Read the model definition and answer for the solid it produces. Units are mm, in the model's axes. Round coordinates to 2 decimals unless told otherwise and drop trailing zeros. Write each loop counter-clockwise with the first axis right and the second up, starting at its lowest first coordinate (ties: lowest second). Pieces come first, ordered by that corner, then holes. Notation, with made-up numbers: (49.25, 74.25) -> (91.25, 74.25) arc R25 ccw to (91.25, 94.25) -> close; hole circle Ø8 at (46, -26.75). An arc over 180 degrees is marked (long way). Return JSON: item names as keys, results as strings. Group by question number.
(1) A cutting plane is placed at A-A on y = 0. Give the vertices of the cut face in (x, z), then the cut area to 3 significant figures.
(2) Given pin 1 (1.2 mm diameter, centred on y = -22.5, z = 16, fed in from -X); pin 2 (3 mm diameter, centred on y = 0, z = 23, fed in from +X); pin 3 (0.6 mm diameter, centred on x = 0, y = -27, fed in from -Z); pin 4 (0.8 mm diameter, centred on x = 0, z = 3.5, fed in from -Y), each flat-ended and moving along its own axis, determine where each tip first touches the part or whether it passes through.
(3) A cutting plane is placed at B-B on z = 16. Give the vertices of the cut face in (x, y).
(4) A cutting plane is placed at C-C on z = 12.8. Give the vertices of the cut face in (x, y), then the cut area to 3 significant figures.
(5) Straight lines are drawn through the part: line 1 (Z direction, x = -0.3, y = 0); line 2 (Y direction, x = -0.1, z = 14); line 3 (Y direction, x = 0.35, z = 20). For each, find the intervals that lie inside material, in ascending order.
(6) A cutting plane is placed at D-D on x = 0.5. State how many separate pieces and enclosed holes the cut face has, then the cut area to 3 significant figures.
```python
from build123d import *

# Parameters (mm, degrees)
F0_R     = 1
F1_DEPTH = 0.75


# Not quite as in the source:
# - ends of sketch curves that miss each other by under 0.0002 mm in the source are joined
# - a feature names something its author has since deleted; it is built from what else it names


with BuildPart() as f1:
    # F0 (on Right) → F1 (new body, symmetric)
    with BuildSketch(Plane.YZ):
        with BuildLine():
            Line((-22.3, -0.8), (-22.3, 6.504902432))
            ThreePointArc((-22.3, 6.504902432), (-22.2756666333, 6.9975905219), (-22.2029033785, 7.4854831077))
            Line((-22.2029033785, 7.4854831077), (-19.9823303189, 18.5883484054))
            ThreePointArc((-19.9823303189, 18.5883484054), (-18.9425550087, 20.320026424), (-17.0405882918, 21))
            Line((-17.0405882918, 21), (12.8226720923, 21))
            ThreePointArc((12.8226720923, 21), (14.5974500424, 20.4187110675), (15.6844554724, 18.9001088187))
            Line((15.6844554724, 18.9001088187), (21, 2))
            Line((21, 2), (22.3, 2))
            ThreePointArc((22.3, 2), (22.4414213562, 1.9414213562), (22.5, 1.8))
            Line((22.5, 1.8), (22.5, 0.2))
            ThreePointArc((22.5, 0.2), (22.4414213562, 0.0585786438), (22.3, 0))
            Line((22.3, 0), (20.2, 0))
            ThreePointArc((20.2, 0), (20.0585786438, -0.0585786438), (20, -0.2))
            Line((20, -0.2), (20, -1.8))
            ThreePointArc((20, -1.8), (20.0585786438, -1.9414213562), (20.2, -2))
            Line((20.2, -2), (23.8107259146, -2))
            ThreePointArc((23.8107259146, -2), (25.2243140233, -1.4148387396), (25.8107251326, -0.001768659))
            ThreePointArc((25.8107251326, -0.001768659), (25.8107257191, -0.0008843296), (25.8107259146, 0))
            ThreePointArc((25.8107259146, 0), (25.8076938609, 0.0370492941), (25.799207863, 0.0732404086))
            Line((25.799207863, 0.0732404086), (19.059851332, 21.5001813645))
            ThreePointArc((19.059851332, 21.5001813645), (17.2481756153, 24.0311851125), (14.2902123652, 25))
            Line((14.2902123652, 25), (-13.6493669984, 25))
            ThreePointArc((-13.6493669984, 25), (-14.5478772467, 25.0813945743), (-15.4171339514, 25.3229282665))
            Line((-15.4171339514, 25.3229282665), (-21.5261195006, 27.6319077703))
            ThreePointArc((-21.5261195006, 27.6319077703), (-22.6761929546, 27.9165348126), (-23.8609482061, 27.9225760631))
            ThreePointArc((-23.8609482061, 27.9225760631), (-34.3671649706, 17.7805604622), (-27.3, 5.0018183321))
            Line((-27.3, 5.0018183321), (-27.3, 2))
            Line((-27.3, 2), (-26.5, 2))
            ThreePointArc((-26.5, 2), (-26.3585786438, 1.9414213562), (-26.3, 1.8))
            Line((-26.3, 1.8), (-26.3, -0.8))
            ThreePointArc((-26.3, -0.8), (-26.2414213562, -0.9414213562), (-26.1, -1))
            Line((-26.1, -1), (-22.5, -1))
            ThreePointArc((-22.5, -1), (-22.3585786438, -0.9414213562), (-22.3, -0.8))
        make_face()
        with Locations((19.6997005895, 12.8)):
            Circle(F0_R, mode=Mode.SUBTRACT)
        with BuildLine():
            Line((-23.5830994757, 20.9805806757), (-26.1667940449, 8.0621078301))
            ThreePointArc((-26.1667940449, 8.0621078301), (-26.4540531191, 7.7032432499), (-26.9129154865, 7.7305725477))
            ThreePointArc((-26.9129154865, 7.7305725477), (-31.2579507019, 17.6226927508), (-23.3162298506, 24.9481581324))
            ThreePointArc((-23.3162298506, 24.9481581324), (-22.308062771, 24.4249028415), (-22.4394560446, 23.2966596198))
            ThreePointArc((-22.4394560446, 23.2966596198), (-23.1634230366, 22.2137470973), (-23.5830994757, 20.9805806757))
        make_face(mode=Mode.SUBTRACT)
        with Locations((-22.5, 16)):
            Circle(F0_R, mode=Mode.SUBTRACT)
        with Locations((0, 23)):
            Circle(F0_R, mode=Mode.SUBTRACT)
        with Locations((16, 22.1668636565)):
            Circle(F0_R, mode=Mode.SUBTRACT)
    extrude(amount=F1_DEPTH, both=True)


solid = f1.part
```
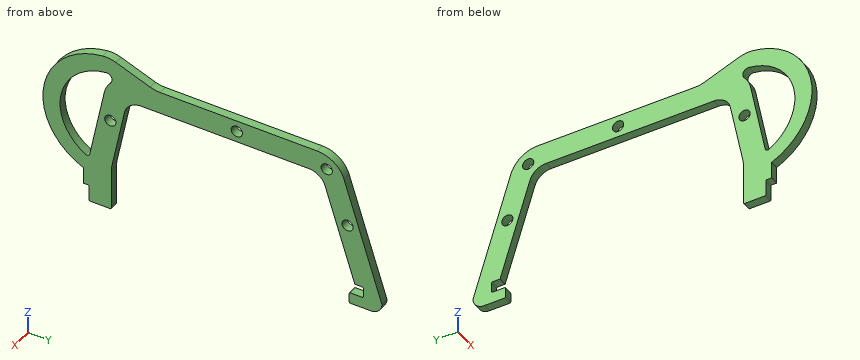
Checks:
{
 "1": {"outline": "(-0.75, 21) -> (0.75, 21) -> (0.75, 22) -> (-0.75, 22) -> close; (-0.75, 24) -> (0.75, 24) -> (0.75, 25) -> (-0.75, 25) -> close", "area": "3.00 mm^2"},
 "2": {"pin 1": "passes through", "pin 2": "stops at x = 0.75", "pin 3": "stops at z = 2", "pin 4": "stops at y = -27.3"},
 "3": {"outline": "(-0.75, -34.5) -> (0.75, -34.5) -> (0.75, -31.45) -> (-0.75, -31.45) -> close; (-0.75, -24.58) -> (0.75, -24.58) -> (0.75, -23.5) -> (-0.75, -23.5) -> close; (-0.75, -21.5) -> (0.75, -21.5) -> (0.75, -20.5) -> (-0.75, -20.5) -> close; (-0.75, 16.6) -> (0.75, 16.6) -> (0.75, 20.79) -> (-0.75, 20.79) -> close"},
 "4": {"outline": "(-0.75, -34.07) -> (0.75, -34.07) -> (0.75, -30.98) -> (-0.75, -30.98) -> close; (-0.75, -25.22) -> (0.75, -25.22) -> (0.75, -21.14) -> (-0.75, -21.14) -> close; (-0.75, 17.6) -> (0.75, 17.6) -> (0.75, 18.7) -> (-0.75, 18.7) -> close; (-0.75, 20.7) -> (0.75, 20.7) -> (0.75, 21.8) -> (-0.75, 21.8) -> close", "area": "14.0 mm^2"},
 "5": {"line 1": "z = 21 to 22, 24 to 25", "line 2": "y = -34.33 to -31.29, -24.98 to -20.9, 17.23 to 21.42", "line 3": "y = -33.81 to -30.41, -23.78 to -19.28, 15.06 to 19.53"},
 "6": {"separate pieces": "1", "enclosed holes": "5", "area": "440 mm^2"}
}
